Read the model definition and answer for the solid it produces. Units are mm, in the model's axes. A direction names the side the tool comes from. Give positions to 0.01 mm unless a question says otherwise; leave off trailing zeros. Loops run counter-clockwise (first coordinate to the right, second up) from the corner with the lowest first, then second, coordinate; pieces in that order, holes last.
(1) Find section C-C, the plane y = 54. Write down the section's boundary in (x, z).
(2) Find section A-A, the plane z = 45.5. Write down the section's boundary in (x, y), then the cut area to 3 significant figures.
(3) Which of the six approach directions +Z, -Z, +X, -X, +Y, -Y give full straight-line access (tool end or side, diameter ignored) to faces 1 (the face through (997, 0, 52)), 2 (the face through (997, 146.05, 51))?
(4) Determine the mould class of faces 3 (the face through (997, 75, 95.25)), 4 (the face through (997, 75, 101.6)), 5 (the face through (997, 152.4, 52)), 6 (the face through (997, 6.35, 50)) for opening direction Y: pulls with the +Y half, pulls with the -Y half, needs draft (parallel to the pull), parting line crosses it, or undercut.
(5) Find section B-B, the plane x = 788. Write down the section's boundary in (y, z).
(6) Straight lines are drawn through the part: probe 1 along Z at (x, y) = (1164.5, 89.5); probe 2 along Y at (x, z) = (923, 31.5); probe 3 along Z at (x, y) = (645.5, 11.5). For each, find the intervals that lie inside material, in ascending order.
```python
from build123d import *

# Parameters (mm, degrees)
SKETCH1_W           = 101.6
SKETCH1_H           = 152.4
BOSS_EXTRUDE1_DEPTH = 2022.623564854
FILLET1_R           = 1


with BuildPart() as part:
    # Sketch1 → Boss-Extrude1 (new body)
    with BuildSketch(Plane(origin=(0, 0, 0), x_dir=(0, 0, -1), z_dir=(1, 0, 0))):
        with Locations((-50.8, 76.2)):
            Rectangle(SKETCH1_W, SKETCH1_H)
        with BuildLine():
            Line((-95.25, 12.7), (-95.25, 139.7))
            ThreePointArc((-95.25, 139.7), (-93.390128061, 144.190128061), (-88.9, 146.05))
            Line((-88.9, 146.05), (-12.7, 146.05))
            ThreePointArc((-12.7, 146.05), (-8.209871939, 144.190128061), (-6.35, 139.7))
            Line((-6.35, 139.7), (-6.35, 12.7))
            ThreePointArc((-6.35, 12.7), (-8.209871939, 8.209871939), (-12.7, 6.35))
            Line((-12.7, 6.35), (-88.9, 6.35))
            ThreePointArc((-88.9, 6.35), (-93.390128061, 8.209871939), (-95.25, 12.7))
        make_face(mode=Mode.SUBTRACT)
    extrude(amount=BOSS_EXTRUDE1_DEPTH)

    # Fillet1
    fillet1_edges = [part.edges().sort_by_distance(p)[0] for p in [
        (2022.623564854, 76.2, 101.6),
        (2022.623564854, 0, 50.8),
        (0, 8.209871939, 93.390128061),
        (0, 6.35, 50.8),
        (0, 8.209871939, 8.209871939),
        (0, 76.2, 6.35),
        (0, 144.190128061, 8.209871939),
        (0, 146.05, 50.8),
        (0, 144.190128061, 93.390128061),
        (0, 76.2, 95.25),
        (2022.623564854, 8.209871939, 93.390128061),
        (2022.623564854, 6.35, 50.8),
        (2022.623564854, 8.209871939, 8.209871939),
        (2022.623564854, 76.2, 6.35),
        (2022.623564854, 144.190128061, 8.209871939),
        (2022.623564854, 146.05, 50.8),
        (2022.623564854, 144.190128061, 93.390128061),
        (2022.623564854, 76.2, 95.25),
        (2022.623564854, 76.2, 0),
        (0, 0, 50.8),
        (0, 76.2, 101.6),
        (0, 152.4, 50.8),
        (0, 76.2, 0),
        (2022.623564854, 152.4, 50.8),
    ]]
    fillet(fillet1_edges, radius=FILLET1_R)


solid = part.part
```
Entries:
1. outline: (0, 1) arc R1 ccw to (1, 0) - (2021.62, 0) arc R1 ccw to (2022.62, 1) - (2022.62, 5.35) arc R1 ccw to (2021.62, 6.35) - (1, 6.35) arc R1 ccw to (0, 5.35) - close; (0, 96.25) arc R1 ccw to (1, 95.25) - (2021.62, 95.25) arc R1 ccw to (2022.62, 96.25) - (2022.62, 100.6) arc R1 ccw to (2021.62, 101.6) - (1, 101.6) arc R1 ccw to (0, 100.6) - close
2. outline: (0, 1) arc R1 ccw to (1, 0) - (2021.62, 0) arc R1 ccw to (2022.62, 1) - (2022.62, 5.35) arc R1 ccw to (2021.62, 6.35) - (1, 6.35) arc R1 ccw to (0, 5.35) - close; (0, 147.05) arc R1 ccw to (1, 146.05) - (2021.62, 146.05) arc R1 ccw to (2022.62, 147.05) - (2022.62, 151.4) arc R1 ccw to (2021.62, 152.4) - (1, 152.4) arc R1 ccw to (0, 151.4) - close
2. area: 25,700 mm2
3. face 1: +Z, -Z, +X, -X, -Y
3. face 2: +X, -X
4. face 3: undercut
4. face 4: needs draft
4. face 5: pulls with the +Y half
4. face 6: undercut
5. outline: (0, 0) - (152.4, 0) - (152.4, 101.6) - (0, 101.6) - close; hole (6.35, 12.7) arc R6.35 ccw to (12.7, 6.35) - (139.7, 6.35) arc R6.35 ccw to (146.05, 12.7) - (146.05, 88.9) arc R6.35 ccw to (139.7, 95.25) - (12.7, 95.25) arc R6.35 ccw to (6.35, 88.9) - close
6. probe 1: z = 0 to 6.35, 95.25 to 101.6
6. probe 2: y = 0 to 6.35, 146.05 to 152.4
6. probe 3: z = 0 to 6.46, 95.14 to 101.6
